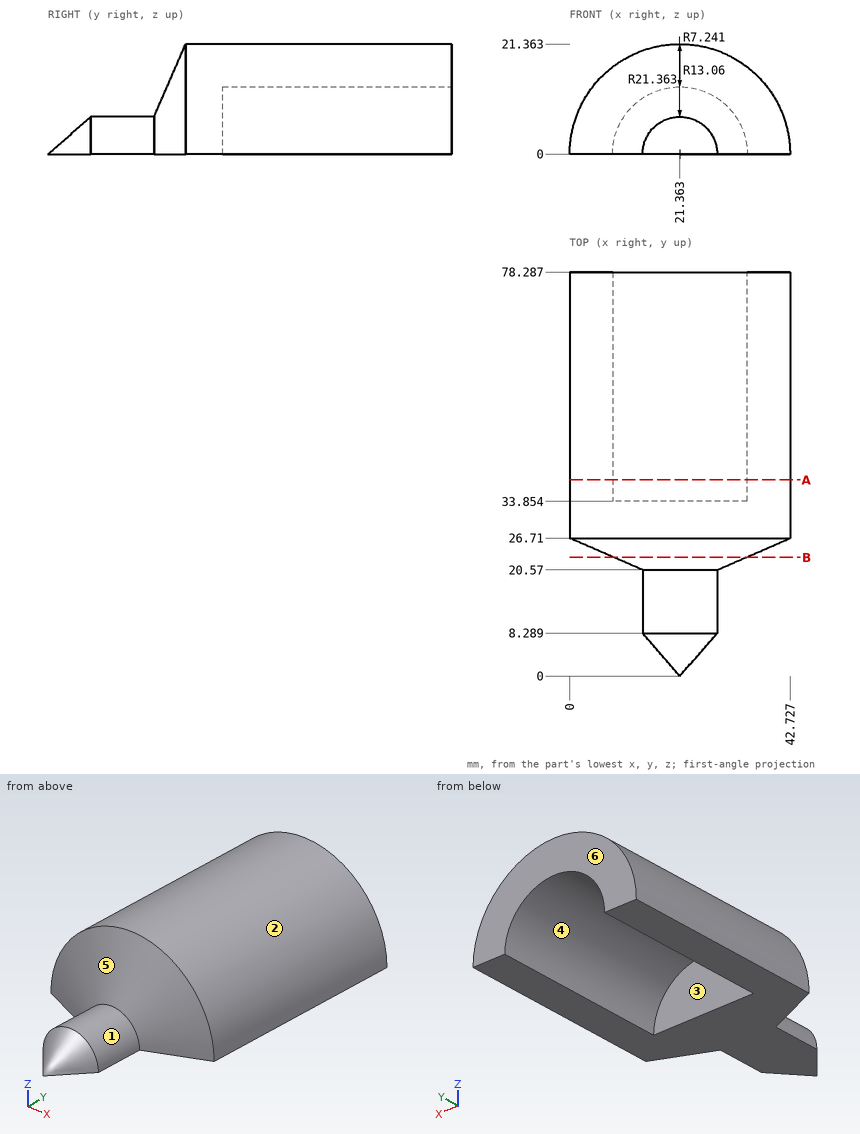
Part print with two shaded views. Sizes in mm from the minimum x, y, z corner. A direction names the side the tool comes from. Round coordinates to 2 decimals unless told otherwise and drop trailing zeros. Loops run counter-clockwise (first coordinate to the right, second up) from the corner with the lowest first, then second, coordinate; pieces in that order, holes last.
Item 1: Saw through at B-B (y = 23). List the corners of the cut face in (x, z) (1 decimal).
Item 2: Which spindle directions (+Z, -Z, +X, -X, +Y, -Y) get a long thin tool onto all of the face, cutting with end or side? Do the marked faces 1, 2 and 3. Say none if no direction does.
Item 3: Drill centre lines: line 1 along X through (y, z) = (55.5, 2.5) (1 decimal); line 2 along X through (y, z) = (56, 6.5) (1 decimal); line 3 along Y through (x, z) = (23, 5.5) (1 decimal). Where is each one in solid material? Low to high.
Item 4: Two-plate mould, pull along X, no slides. Class the marked faces 4, 5 and 6: released by +X, released by -X, zero draft, split by the parting line, or undercut.
Item 5: Pin check, flat tips, straight feed: P1, Ø5, axis at x = 32, z = 18.5, coming from the -Y side; P2, Ø6, axis at x = 26, z = 12.5, coming from the -Y side; P3, Ø3, axis at x = 32, y = 29, coming from the +Z side. Stop position of each tip, or through.
Item 6: Saw through at A-A (y = 38). List the corners of the cut face in (x, z), then the cut area to 3 significant figures.
Worked answers:
1. outline: (8.5, 0) - (34.2, 0) arc R12.8 ccw to start
2. face 1: +Z, -Y
2. face 2: +Z, +Y, -Y
2. face 3: -Z, +Y
3. line 1: x = 0.1 to 8.5, 34.2 to 42.6
3. line 2: x = 1 to 10, 32.7 to 41.7
3. line 3: y = 6.6 to 33.9
4. face 4: undercut
4. face 5: split by the parting line
4. face 6: zero draft
5. P1: stops at y = 25.61
5. P2: stops at y = 21.91
5. P3: stops at z = 19.31
6. outline: (0, 0) - (8.3, 0) arc R13.06 cw to (34.42, 0) - (42.73, 0) arc R21.36 ccw to start
6. area: 449 mm2
